Check sheet for the modelled part. Datum: model origin and axes. Units: mm. Give positions to 0.01 mm unless a question says otherwise; leave off trailing zeros. Write each loop counter-clockwise with the first axis right and the second up, starting at its lowest first coordinate (ties: lowest second). Pieces come first, ordered by that corner, then holes. Notation, with made-up numbers: M 42.25,41.5 L 58.25,41.5 A31 cw 58.25,77.5 Z; hole C -1.5,-17.5 d7. An arc over 180 degrees is marked long. Write item = value, one per line. Start each with the question number.
1) Cross-section at B-B, the plane x = 38. Record the cut outline in (y, z).
2) Scan lines: line 1 along Z through (x, y) = (48.5, 732.5); line 2 along Y through (x, z) = (46, -347). Record each from-to range of solid material in increasing order. Write a range as [from, to].
3) Cross-section at C-C, the plane z = -414.5. Record the cut outline in (x, y).
4) Go/stop test with flat-tipped pins: pin 1 (8 mm diameter, centred on x = 35.5, z = -387.5, fed in from +Y); pin 2 (12 mm diameter, centred on y = 463, z = -423, fed in from -X); pin 3 (4 mm diameter, centred on x = 30.5, z = -75, fed in from -Y). Record where each tip stops, or that it passes through.
5) Cross-section at A-A, the plane y = 750. Record the cut outline in (x, z).
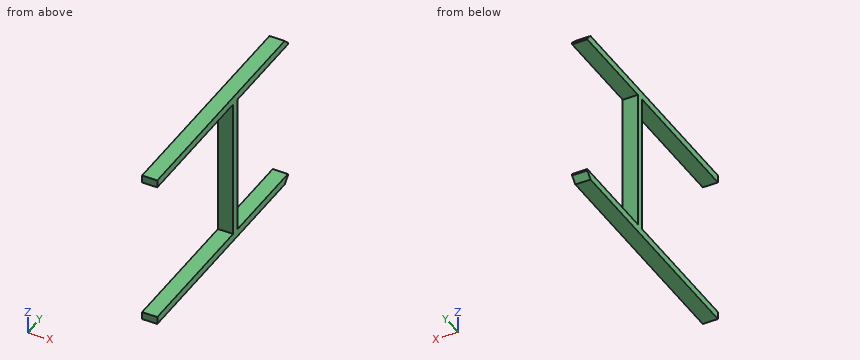
```python
from build123d import *

# Parameters (mm, degrees)
CROQUIS2_W                = 50.8
CROQUIS2_H                = 25.4
SALIENTE_EXTRUIR1_DEPTH   = 800
SALIENTE_EXTRUIR1_2_DEPTH = 800
CROQUIS3_W                = 50.8
CROQUIS3_H                = 25.4
SALIENTE_EXTRUIR2_DEPTH   = 474
CHAFL_N1_SIZE             = 20


with BuildPart() as part:
    # Croquis2 → Saliente-Extruir1 (new body)
    with BuildSketch(Plane(origin=(0, 0, 0), x_dir=(1, 0, 0), z_dir=(0, 1, 0))):
        with Locations((25.4, -12.7)):
            Rectangle(CROQUIS2_W, CROQUIS2_H)
    extrude(amount=SALIENTE_EXTRUIR1_DEPTH)



with BuildPart() as body_2:
    # Croquis2 → Saliente-Extruir1 2 (new body)
    with BuildSketch(Plane(origin=(0, 0, 0), x_dir=(1, 0, 0), z_dir=(0, 1, 0))):
        with Locations((25.4, 486.7)):
            Rectangle(CROQUIS2_W, CROQUIS2_H)
    extrude(amount=SALIENTE_EXTRUIR1_2_DEPTH)


with BuildPart() as part_1:
    add(part.part)

    add(body_2.part)  # Saliente-Extruir2 merges body 2
    # Croquis3 → Saliente-Extruir2 (add)
    with BuildSketch(Plane.XY.offset(-474)):
        with Locations((25.4, 477.3)):
            Rectangle(CROQUIS3_W, CROQUIS3_H)
    extrude(amount=SALIENTE_EXTRUIR2_DEPTH)

    # Chaflán1
    chafl_n1_edges = [part_1.edges().sort_by_distance(p)[0] for p in [
        (25.4, 800, 25.4),
        (25.4, 800, -499.4),
    ]]
    chamfer(chafl_n1_edges, length=CHAFL_N1_SIZE)


solid = part_1.part
```
Reply:
q1.outline = M 0,-499.4 L 780,-499.4 L 800,-479.4 L 800,-474 L 490,-474 L 490,0 L 800,0 L 800,5.4 L 780,25.4 L 0,25.4 L 0,0 L 464.6,0 L 464.6,-474 L 0,-474 Z
q2.line_1 = [-499.4, -474], [0, 25.4]
q2.line_2 = [464.6, 490]
q3.outline = M 0,464.6 L 50.8,464.6 L 50.8,490 L 0,490 Z
q4.pin_1 = 490
q4.pin_2 = 0
q4.pin_3 = 464.6
q5.outline = M 0,-499.4 L 50.8,-499.4 L 50.8,-474 L 0,-474 Z; M 0,0 L 50.8,0 L 50.8,25.4 L 0,25.4 Z
